Model file for the job. Use its own axes, mm. Round coordinates to 2 decimals unless told otherwise and drop trailing zeros. Loops run counter-clockwise (first coordinate to the right, second up) from the corner with the lowest first, then second, coordinate; pieces in that order, holes last. Notation, with made-up numbers: M -3.75,72 L 40.25,72 A29 ccw 40.25,95 Z; hole C 73,-34 d7. An arc over 180 degrees is marked long. Answer in a Markdown table with one row per item.
from build123d import *

# Parameters (mm, degrees)
EXTRUDE1_DEPTH = 609.6


with BuildPart() as part:
    # Sketch1 → Extrude1 (new body)
    with BuildSketch(Plane.XY):
        with BuildLine():
            Line((2.9718, 33.528), (-2.9718, 33.528))
            ThreePointArc((-2.9718, 33.528), (-3.739183777, 33.43386792), (-4.46106492, 33.157053316))
            Line((-4.46106492, 33.157053316), (-26.56126623, 21.419382585))
            ThreePointArc((-26.56126623, 21.419382585), (-28.56180679, 19.522269649), (-29.2989, 16.8656))
            Line((-29.2989, 16.8656), (-29.2989, -9.652))
            ThreePointArc((-29.2989, -9.652), (-28.394883916, -12.568389957), (-25.999830769, -14.462141759))
            ThreePointArc((-25.999830769, -14.462141759), (-22.985772925, -15.549597701), (-19.926426205, -16.502227094))
            ThreePointArc((-19.926426205, -16.502227094), (-17.139768103, -15.98665549), (-15.875, -13.450587845))
            Line((-15.875, -13.450587845), (-15.875, -10.240713335))
            ThreePointArc((-15.875, -10.240713335), (-15.971069561, -9.465592471), (-16.253464474, -8.737379023))
            ThreePointArc((-16.253464474, -8.737379023), (0, 18.4531), (16.253464474, -8.737379023))
            ThreePointArc((16.253464474, -8.737379023), (15.971069561, -9.465592471), (15.875, -10.240713335))
            Line((15.875, -10.240713335), (15.875, -13.450587845))
            ThreePointArc((15.875, -13.450587845), (17.139768103, -15.98665549), (19.926426205, -16.502227094))
            ThreePointArc((19.926426205, -16.502227094), (22.985772925, -15.549597701), (25.999830769, -14.462141759))
            ThreePointArc((25.999830769, -14.462141759), (28.394883916, -12.568389957), (29.2989, -9.652))
            Line((29.2989, -9.652), (29.2989, 16.8656))
            ThreePointArc((29.2989, 16.8656), (28.56180679, 19.522269649), (26.56126623, 21.419382585))
            Line((26.56126623, 21.419382585), (4.46106492, 33.157053316))
            ThreePointArc((4.46106492, 33.157053316), (3.739183777, 33.43386792), (2.9718, 33.528))
        make_face()
    extrude(amount=-EXTRUDE1_DEPTH)


solid = part.part
1. Pin check, flat tips, straight feed: pin 1 (2.5 mm diameter, centred on y = -11.5, z = -397, fed in from -X); pin 2 (12 mm diameter, centred on x = -8.5, y = -10.5, fed in from +Z); pin 3 (4 mm diameter, centred on x = -22.5, z = -481.5, fed in from +Y); pin 4 (1.5 mm diameter, centred on x = 23, z = -120, fed in from +Y). Stop position of each tip, or through.
Verdict:
| item | result |
|---|---|
| pin 1 | stops at x = -29.26 |
| pin 2 | passes through |
| pin 3 | stops at y = 24.64 |
| pin 4 | stops at y = 23.71 |
2. Wall check: probe 1 along X at (y, z) = (-0.5, -365.5); probe 2 along Y at (x, z) = (-16.5, -182.5). Give the ranges that are in metal, low to high.
Verdict:
| item | result |
|---|---|
| probe 1 | x = -29.3 to -18.45, 18.45 to 29.3 |
| probe 2 | y = -15.34 to -8.26, 8.26 to 26.76 |
3. Saw through at B-B (z = -366). Write the cut outline in (x, y) (3 decimals).
Verdict:
| item | result |
|---|---|
| outline | M -29.299,-9.652 A5.156 ccw -26,-14.462 A72.187 ccw -19.926,-16.502 A3.175 ccw -15.875,-13.451 L -15.875,-10.241 A3.175 ccw -16.253,-8.737 A18.453 cw long 16.253,-8.737 A3.175 ccw 15.875,-10.241 L 15.875,-13.451 A3.175 ccw 19.926,-16.502 A72.187 ccw 26,-14.462 A5.156 ccw 29.299,-9.652 L 29.299,16.866 A5.156 ccw 26.561,21.419 L 4.461,33.157 A3.175 ccw 2.972,33.528 L -2.972,33.528 A3.175 ccw -4.461,33.157 L -26.561,21.419 A5.156 ccw -29.299,16.866 Z |
4. Saw through at A-A (y = 0). Write the cut outline in (x, z).
Verdict:
| item | result |
|---|---|
| outline | M -29.3,-609.6 L -18.45,-609.6 L -18.45,0 L -29.3,0 Z; M 18.45,-609.6 L 29.3,-609.6 L 29.3,0 L 18.45,0 Z |
5. Mould opens along Y. For faces 1 (the flat face through (15.666, 27.206, -300.533)), 2 (the cylindrical face through (-0.533, 18.445, -300.533)), 3 (the flat face through (0, 20, -609.6)) say: +Y half, -Y half, draft (parallel to the pull), parting line (faces both ways), or undercut.
Verdict:
| item | result |
|---|---|
| face 1 | +Y half |
| face 2 | undercut |
| face 3 | draft |
